Input: part model. Units: mm. Frame: model coordinates. A direction names the side the tool comes from. Give positions to 0.01 mm unless a question says otherwise; leave off trailing zeros. Order: outer loops, then holes, each group sorted by start corner. A loop starts at its lowest first (then second) coordinate and runs counter-clockwise, first axis right, second up. Notation, with made-up numbers: (85.5, 13.5) - (114.5, 13.5) arc R15 ccw to (114.5, 20.5) - close; hole circle Ø2 at (-21, -4). An arc over 180 degrees is marked (long way). Answer in a Markdown table with one row per item. Add a question column.
1. Section query D-D on y = -2.75. Return loops of the section in (x, z), and give its area (3 significant figures).
2. Access query for faces 5 (the face through (-2, -3, 5)), 6 (the face through (-5.3, -2.6, 5.1)). Directions: +Z, -Z, +X, -X, +Y, -Y. A direction counts if a zero-diameter tool reaches every point of the face in a straight line with its end or side. Return the directions, or none.
3. Section query B-B on y = -5. Return loops of the section in (x, z).
4. Ray query, line 1 (X direction, y = -1.55, z = 5); line 2 (X direction, y = -6.75, z = 8.75); line 3 (Y direction, x = -1, z = 8.75). Return the intervals inside material, ascending. Write a range as [from, to].
5. Mould query, pull axis X, two halves, no side actions, for faces 1 (the face through (-0.61, -1.48, 6.48)), 2 (the face through (-8, -4, 5)), 3 (the face through (2, 0, 5)), 4 (the face through (5.4, -2.7, 5.1)). Classes: released by +X, released by -X, zero draft, split by the parting line, or undercut.
6. Section query A-A on x = 0. Return loops of the section in (y, z), and give its area (3 significant figures).
7. Section query C-C on z = 4.75. Return loops of the section in (x, y), and give its area (3 significant figures).
```python
from build123d import *

# Parameters (mm, degrees)
EXTRUDE_1_DEPTH     = 10
SKETCH_2_R          = 1.6
CUT_EXTRUDE_1_DEPTH = 16.652475842
SKETCH_5_R          = 0.5
CUT_EXTRUDE_2_DEPTH = 16.652475842


with BuildPart() as part:
    # 草图1 → 凸台-拉伸1 (new body)
    with BuildSketch(Plane.XY):
        Polygon((0, 0), (-8, 0), (-8, -9), (-5, -9), (-5, -3), (5, -3), (5, -9), (8, -9), (8, 0), align=None)
    extrude(amount=EXTRUDE_1_DEPTH)

    # 草图2 → 切除-拉伸1 (cut, through all)
    with BuildSketch(Plane(origin=(0, 0, 0), x_dir=(1, 0, 0), z_dir=(0, 1, 0))):
        with Locations(Location((0, -5, 0), (0, 0, 270))):
            Circle(SKETCH_2_R)
    extrude(amount=-CUT_EXTRUDE_1_DEPTH, mode=Mode.SUBTRACT)

    # 草图5 → 切除-拉伸2 (cut, through all)
    with BuildSketch(Plane.XY.offset(10)):
        with Locations((-5, -3)):
            Circle(SKETCH_5_R)
        with Locations((5, -3)):
            Circle(SKETCH_5_R)
    extrude(amount=-CUT_EXTRUDE_2_DEPTH, mode=Mode.SUBTRACT)


solid = part.part
```
Answer:
| question | item | result |
|---|---|---|
| 1 | outline | (-8, 0) - (-5.43, 0) - (-5.43, 10) - (-8, 10) - close; (-4.57, 0) - (4.57, 0) - (4.57, 10) - (-4.57, 10) - close; (5.43, 0) - (8, 0) - (8, 10) - (5.43, 10) - close; hole circle Ø3.2 at (0, 5) |
| 1 | area | 135 mm² |
| 2 | face 5 | +Z, -Z, -Y |
| 2 | face 6 | +Z, -Z |
| 3 | outline | (-8, 0) - (-5, 0) - (-5, 10) - (-8, 10) - close; (5, 0) - (8, 0) - (8, 10) - (5, 10) - close |
| 4 | line 1 | x = [-8, -1.6], [1.6, 8] |
| 4 | line 2 | x = [-8, -5], [5, 8] |
| 4 | line 3 | y = [-3, 0] |
| 5 | face 1 | undercut |
| 5 | face 2 | released by -X |
| 5 | face 3 | zero draft |
| 5 | face 4 | undercut |
| 6 | outline | (-3, 0) - (0, 0) - (0, 3.4) - (-3, 3.4) - close; (-3, 6.6) - (0, 6.6) - (0, 10) - (-3, 10) - close |
| 6 | area | 20.4 mm² |
| 7 | outline | (-8, -9) - (-5, -9) - (-5, -3.5) arc R0.5 cw (long way) to (-4.5, -3) - (-1.58, -3) - (-1.58, 0) - (-8, 0) - close; (1.58, -3) - (4.5, -3) arc R0.5 cw (long way) to (5, -3.5) - (5, -9) - (8, -9) - (8, 0) - (1.58, 0) - close |
| 7 | area | 73.3 mm² |
